Geometry check sheet. Reference: the model listing, model coordinates, mm. Face numbers are marked on the shaded views. A direction names the side the tool comes from. Give positions to 0.01 mm unless a question says otherwise; leave off trailing zeros. Loops run counter-clockwise (first coordinate to the right, second up) from the corner with the lowest first, then second, coordinate; pieces in that order, holes last.
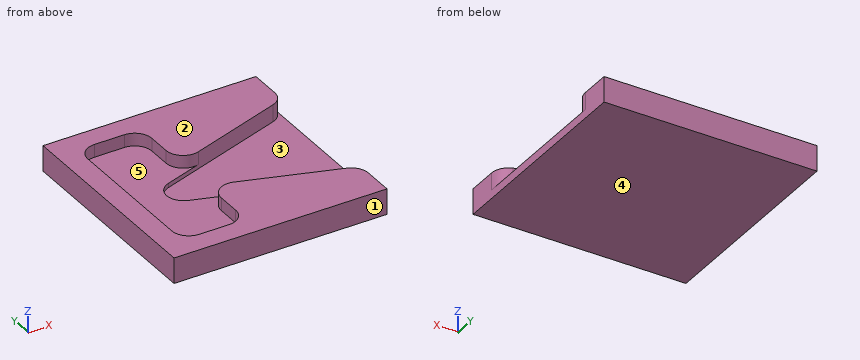
```python
from build123d import *

# Parameters (mm, degrees)
F0_W     = 100
F0_H     = 100
F1_DEPTH = 12
F2_W     = 30
F2_H     = 80
F3_DEPTH = 6
F5_DEPTH = 8
F6_R     = 8


with BuildPart() as f1:
    # F0 (on Top) → F1 (new body)
    with BuildSketch(Plane.XY):
        with Locations((50, 50)):
            Rectangle(F0_W, F0_H)
    extrude(amount=F1_DEPTH)

    # F2 (on face) → F3 (cut)
    with BuildSketch(Plane.XY.offset(12)):
        with Locations((25, 50)):
            Rectangle(F2_W, F2_H)
    extrude(amount=-F3_DEPTH, mode=Mode.SUBTRACT)

    # F4 (on face) → F5 (cut)
    with BuildSketch(Plane.XY.offset(12)):
        Polygon((100, 80), (40, 60), (40, 40), (100, 20), align=None)
        Polygon((40, 60), (10, 50), (40, 40), align=None)
    extrude(amount=-F5_DEPTH, mode=Mode.SUBTRACT)

    # F6
    f6_edges = [f1.edges().sort_by_distance(p)[0] for p in [
        (10, 50, 5),
        (10, 90, 9),
        (10, 10, 9),
        (40, 90, 9),
        (40, 10, 9),
        (100, 20, 8),
        (100, 80, 8),
        (40, 60, 9),
        (40, 40, 9),
    ]]
    fillet(f6_edges, radius=F6_R)


solid = f1.part
```
1) Sectioned sample at C-C on z = 8.5. Enter the section's corners in (x, y).
2) Depth check by flat-ended pin: P1, Ø1.8, axis at y = 50, z = 10.5, coming from the +X side; P2, Ø2, axis at x = 39.5, y = 49, coming from the +Z side; P3, Ø1.5, axis at x = 73, z = 8.5, coming from the -Y side; P4, Ø20.5, axis at x = 21, y = 64, coming from the +Z side. Enter the tip coordinate at first touch or a pass-through.
3) Tool access check on the marked faces 4 and 5. Record the directions out of +Z, -Z, +X, -X, +Y, -Y that give a thin tool (end or side, any length) a straight path to the whole face; none if there is none.
4) Mould release check, pull along Y, two halves, no side actions. Record for the marked faces 1, 2 and 3: +Y half, -Y half, draft (parallel to the pull), parting line (faces both ways), or undercut.
5) Scan lines: line 1 along Y through (x, z) = (20.5, 9.75); line 2 along Z through (x, y) = (38, 26.5); line 3 along Z through (x, y) = (69, 51). Record each from-to range of solid material in increasing order.
6) Sectioned sample at B-B on y = 23.5. Enter the section's corners in (x, z).
7) Sectioned sample at D-D on y = 47.5. Enter the section's corners in (x, z), plus the area to 3 significant figures.
8) Sectioned sample at A-A on x = 89.5. Enter the section's corners in (y, z), plus the area to 3 significant figures.
Determined:
1. outline: (0, 0) - (100, 0) - (100, 14.23) arc R8 ccw to (94.53, 21.82) - (50.53, 36.49) arc R8 ccw to (40, 28.9) - (40, 18) arc R8 cw to (32, 10) - (18, 10) arc R8 cw to (10, 18) - (10, 82) arc R8 cw to (18, 90) - (32, 90) arc R8 cw to (40, 82) - (40, 71.1) arc R8 ccw to (50.53, 63.51) - (94.53, 78.18) arc R8 ccw to (100, 85.77) - (100, 100) - (0, 100) - close
2. P1: stops at x = 10
2. P2: stops at z = 4
2. P3: stops at y = 0
2. P4: stops at z = 6
3. face 4: -Z, +X, -X, +Y, -Y
3. face 5: +Z
4. face 1: -Y half
4. face 2: draft
4. face 3: undercut
5. line 1: y = 0 to 10, 90 to 100
5. line 2: z = 0 to 6
5. line 3: z = 0 to 4
6. outline: (0, 0) - (100, 0) - (100, 4) - (89.5, 4) - (89.5, 12) - (40, 12) - (40, 6) - (10, 6) - (10, 12) - (0, 12) - close
7. outline: (0, 0) - (100, 0) - (100, 4) - (27.7, 4) - (27.7, 6) - (10, 6) - (10, 12) - (0, 12) - close
7. area: 515 mm2
8. outline: (0, 0) - (100, 0) - (100, 12) - (76.5, 12) - (76.5, 4) - (23.5, 4) - (23.5, 12) - (0, 12) - close
8. area: 776 mm2
